Geometry: final body of the model. Coordinates: model frame, mm. Round coordinates to 2 decimals unless told otherwise and drop trailing zeros. Write item = value, one per line. Start each with the question number.
Item 1: Draft query along Y for faces 1 (the flat face through (215, 74, 0)), 2 (the cylindrical face through (422.98, 47.463, 1.127)). Return one class per face: pulls with the +Y half, pulls with the -Y half, needs draft (parallel to the pull), parting line crosses it, or undercut.
Item 2: First-contact query: pin 1 (5 mm diameter, centred on x = 167.64, y = 91.44, fed in from +Z). Flat tip, straight axial feed; report the tip coordinate or a pass-through.
Item 3: Section A-A (x = 105). Count the separate pieces of the cut face and the enclosed holes in it, plus the area to 3 significant figures.
Item 4: Line query: line 1 (Y direction, x = 269, z = 1.65); line 2 (Y direction, x = 89, z = 0.15); line 3 (X direction, y = 40, z = 0.3). Output: solid intervals per line, ascending. Write a range as from..to.
Autodesk Inventor part; units mm, degrees
ref_plane "YZ Plane" through (0, 0, 0) normal (1, 0, 0) x (0, 1, 0)
ref_plane "XZ Plane" through (0, 0, 0) normal (0, 1, 0) x (-1, 0, 0)
ref_plane "XY Plane" through (0, 0, 0) normal (0, 0, 1) x (1, 0, 0)
sketch "Sketch1" plane through (0, 0, 0) normal (0, 0, 1) x (1, 0, 0)
  line L0 (0, 0) -> (436.118, 0)
  line L1 (436.118, 0) -> (436.118, 101.6)
  line L2 (436.118, 101.6) -> (0, 101.6)
  line L3 (0, 101.6) -> (0, 0)
  circle A0 centre (12.7, 88.9) radius 3.3655
  circle A1 centre (12.7, 50.8) radius 3.3655
  circle A2 centre (12.7, 12.7) radius 3.3655
  circle A3 centre (423.418, 88.9) radius 3.3655
  circle A4 centre (423.418, 50.8) radius 3.3655
  circle A5 centre (423.418, 12.7) radius 3.3655
  circle A6 centre (218.059, 50.8) radius 20.32
  dimension "d0" = 436.118
  dimension "d1" = 101.6
  dimension "d2" = 6.731
  dimension "d3" = 12.7
  dimension "d4" = 12.7
  dimension "d7" = 38.1
  dimension "d10" = 410.718
  dimension "d13" = 12.7
  dimension "d24" = 40.64
  dimension "d25" = 50.8
  dimension "d26" = 218.059
extrude "Extrusion1" add sketch "Sketch1" along normal blind 2.286
sketch "Sketch2" plane through (0, 0, 2.286) normal (0, 0, 1) x (1, 0, 0)
  line L0 (0, 0) -> (436.118, 0)
  line L1 (82.55, 0) -> (133.35, 0)
  line L2 (31.75, 101.6) -> (184.15, 101.6)
  line L3 (133.35, 0) -> (184.15, 101.6)
  line L4 (31.75, 101.6) -> (82.55, 0)
  line L5 (97.1739, 7) -> (117.1739, 7)
  line L6 (117.1739, 7) -> (117.1739, 2)
  line L7 (117.1739, 2) -> (97.1739, 2)
  line L8 (97.1739, 2) -> (97.1739, 7)
  line L9 (133.35, 0) -> (133.35, 62.4863)
  line L10 (97.1739, 14) -> (117.1739, 14)
  line L11 (117.1739, 14) -> (117.1739, 9)
  line L12 (117.1739, 9) -> (97.1739, 9)
  line L13 (97.1739, 9) -> (97.1739, 14)
  line L14 (97.1739, 21) -> (117.1739, 21)
  line L15 (117.1739, 21) -> (117.1739, 16)
  line L16 (117.1739, 16) -> (97.1739, 16)
  line L17 (97.1739, 16) -> (97.1739, 21)
  line L18 (97.1739, 28) -> (117.1739, 28)
  line L19 (117.1739, 28) -> (117.1739, 23)
  line L20 (117.1739, 23) -> (97.1739, 23)
  line L21 (97.1739, 23) -> (97.1739, 28)
  line L22 (97.1739, 35) -> (117.1739, 35)
  line L23 (117.1739, 35) -> (117.1739, 30)
  line L24 (117.1739, 30) -> (97.1739, 30)
  line L25 (97.1739, 30) -> (97.1739, 35)
  line L26 (97.1739, 42) -> (117.1739, 42)
  line L27 (117.1739, 42) -> (117.1739, 37)
  line L28 (117.1739, 37) -> (97.1739, 37)
  line L29 (97.1739, 37) -> (97.1739, 42)
  circle A0 centre (126.2557, 6.2222) radius 3.1623
  circle A1 centre (126.2557, 28) radius 3.1623
  circle A2 centre (126.2557, 49.7778) radius 3.1623
  line L30 (107.95, 0) -> (107.95, -15.6085)
  circle A3 centre (89.6443, 49.7778) radius 3.1623
  circle A4 centre (89.6443, 6.2222) radius 3.1623
  circle A5 centre (89.6443, 28) radius 3.1623
  line L31 (117.1739, 44) -> (97.1739, 44)
  line L32 (97.1739, 44) -> (97.1739, 49)
  line L33 (117.1739, 49) -> (117.1739, 44)
  line L34 (97.1739, 49) -> (117.1739, 49)
  line L35 (117.1739, 51) -> (97.1739, 51)
  line L36 (97.1739, 51) -> (97.1739, 56)
  line L37 (97.1739, 56) -> (117.1739, 56)
  line L38 (117.1739, 56) -> (117.1739, 51)
  circle A6 centre (48.26, 91.44) radius 3.1623
  circle A7 centre (167.64, 91.44) radius 3.1623
  circle A8 centre (48.26, 10.16) radius 3.1623
  circle A9 centre (167.64, 10.16) radius 3.1623
  point P0 (0, 101.6)
  dimension "d37" = 50.8
  dimension "d38" = 152.4
  dimension "d39" = 101.6
  dimension "d40" = 50.8
  dimension "d41" = 20
  dimension "d42" = 5
  dimension "d43" = 2
  dimension "d44" = 7
  dimension "d45" = 6.3246
  dimension "d46" = 6.3246
  dimension "d47" = 6.3246
  dimension "d48" = 14
  dimension "d49" = 56
  dimension "d50" = 6.2222
  dimension "d51" = 6.2222
  dimension "d52" = 28
  dimension "d53" = 6.3246
  dimension "d54" = 6.3246
  dimension "d55" = 34.29
  dimension "d56" = 34.29
  dimension "d57" = 10.16
  dimension "d58" = 10.16
  dimension "d61" = 16.1761
  dimension "d62" = 31.75
  dimension "d112" = 9.0818
  dimension "d113" = 9.0818
  dimension "d114" = 9.0818
  dimension "d115" = 6.3246
  dimension "d116" = 10.16
  dimension "d117" = 34.29
  dimension "d118" = 6.3246
  dimension "d119" = 10.16
  dimension "d120" = 34.29
extrude "Extrusion2" cut sketch "Sketch2" against normal blind 2.286 contours L5 L6 L7 L8 | L10 L11 L12 L13 | L14 L15 L16 L17 | L18 L19 L20 L21 | L22 L23 L24 L25 | L26 L27 L28 L29 | A0 | A1 | A2 | A3 | A4 | A5 | L31 L32 L34 L33 | L35 L36 L37 L38 | A6 | A7 | A8 | A9
sketch "Sketch3" plane through (0, 0, 2.286) normal (0, 0, 1) x (1, 0, 0)
  circle A0 centre (126.2557, 49.7778) radius 3.1623
  line L0 (117.1739, 56) -> (117.1739, 51)
  line L1 (0, 0) -> (436.118, 0)
  line L2 (302.768, 0) -> (353.568, 0)
  line L3 (251.968, 101.6) -> (404.368, 101.6)
  line L4 (353.568, 0) -> (404.368, 101.6)
  line L5 (251.968, 101.6) -> (302.768, 0)
  line L6 (317.3919, 7) -> (337.3919, 7)
  line L7 (337.3919, 7) -> (337.3919, 2)
  line L8 (337.3919, 2) -> (317.3919, 2)
  line L9 (317.3919, 2) -> (317.3919, 7)
  line L10 (353.568, 0) -> (353.568, 62.4863)
  line L11 (317.3919, 14) -> (337.3919, 14)
  line L12 (337.3919, 14) -> (337.3919, 9)
  line L13 (337.3919, 9) -> (317.3919, 9)
  line L14 (317.3919, 9) -> (317.3919, 14)
  line L15 (317.3919, 21) -> (337.3919, 21)
  line L16 (337.3919, 21) -> (337.3919, 16)
  line L17 (337.3919, 16) -> (317.3919, 16)
  line L18 (317.3919, 16) -> (317.3919, 21)
  line L19 (317.3919, 28) -> (337.3919, 28)
  line L20 (337.3919, 28) -> (337.3919, 23)
  line L21 (337.3919, 23) -> (317.3919, 23)
  line L22 (317.3919, 23) -> (317.3919, 28)
  line L23 (317.3919, 35) -> (337.3919, 35)
  line L24 (337.3919, 35) -> (337.3919, 30)
  line L25 (337.3919, 30) -> (317.3919, 30)
  line L26 (317.3919, 30) -> (317.3919, 35)
  line L27 (317.3919, 42) -> (337.3919, 42)
  line L28 (337.3919, 42) -> (337.3919, 37)
  line L29 (337.3919, 37) -> (317.3919, 37)
  line L30 (317.3919, 37) -> (317.3919, 42)
  circle A1 centre (346.4737, 6.2222) radius 3.1623
  circle A2 centre (346.4737, 28) radius 3.1623
  circle A3 centre (346.4737, 49.7778) radius 3.1623
  line L31 (328.168, 0) -> (328.168, -15.6085)
  circle A4 centre (309.8623, 49.7778) radius 3.1623
  circle A5 centre (309.8623, 6.2222) radius 3.1623
  circle A6 centre (309.8623, 28) radius 3.1623
  line L32 (337.3919, 44) -> (317.3919, 44)
  line L33 (317.3919, 44) -> (317.3919, 49)
  line L34 (337.3919, 49) -> (337.3919, 44)
  line L35 (317.3919, 49) -> (337.3919, 49)
  line L36 (337.3919, 51) -> (317.3919, 51)
  line L37 (317.3919, 51) -> (317.3919, 56)
  line L38 (317.3919, 56) -> (337.3919, 56)
  line L39 (337.3919, 56) -> (337.3919, 51)
  circle A7 centre (268.478, 91.44) radius 3.1623
  circle A8 centre (387.858, 91.44) radius 3.1623
  circle A9 centre (268.478, 10.16) radius 3.1623
  circle A10 centre (387.858, 10.16) radius 3.1623
  point P0 (436.118, 101.6)
  dimension "d74" = 50.8
  dimension "d75" = 152.4
  dimension "d76" = 101.6
  dimension "d77" = 50.8
  dimension "d78" = 20
  dimension "d79" = 5
  dimension "d80" = 2
  dimension "d81" = 7
  dimension "d82" = 6.3246
  dimension "d83" = 6.3246
  dimension "d84" = 6.3246
  dimension "d85" = 14
  dimension "d86" = 56
  dimension "d87" = 6.2222
  dimension "d88" = 6.2222
  dimension "d89" = 28
  dimension "d90" = 6.3246
  dimension "d91" = 6.3246
  dimension "d92" = 34.29
  dimension "d93" = 34.29
  dimension "d94" = 10.16
  dimension "d95" = 10.16
  dimension "d98" = 16.1761
  dimension "d99" = 31.75
  dimension "d100" = 9.0818
  dimension "d101" = 9.0818
  dimension "d102" = 9.0818
  dimension "d103" = 9.0818
  dimension "d104" = 6.3246
  dimension "d105" = 10.16
  dimension "d106" = 34.29
  dimension "d107" = 6.3246
  dimension "d108" = 10.16
  dimension "d109" = 34.29
extrude "Extrusion3" cut sketch "Sketch3" against normal blind 6.3246 contours L6 L7 L8 L9 | L11 L12 L13 L14 | L15 L16 L17 L18 | L19 L20 L21 L22 | L23 L24 L25 L26 | L27 L28 L29 L30 | A1 | A2 | A3 | A4 | A5 | A6 | L32 L33 L35 L34 | L36 L37 L38 L39 | A7 | A8 | A9 | A10
equation "\"d26\" = 0.5 * d0"
equation "\"d46\" = d45"
equation "\"d47\" = d46"
equation "\"d50\" = 0.111111 * d49"
equation "\"d51\" = d50"
equation "\"d52\" = 0.5 * d49"
equation "\"d56\" = d55"
equation "\"d58\" = d57"
equation "\"d113\" = d112"
equation "\"d114\" = d112"
equation "\"d116\" = d57"
equation "\"d117\" = d56"
equation "\"d119\" = d58"
equation "\"d120\" = d55"
equation "\"d83\" = d82"
equation "\"d84\" = d83"
equation "\"d87\" = 0.111111 * d86"
equation "\"d88\" = d87"
equation "\"d89\" = 0.5 * d86"
equation "\"d93\" = d92"
equation "\"d95\" = d94"
equation "\"d102\" = d100"
equation "\"d103\" = d100"
equation "\"d105\" = d94"
equation "\"d106\" = d93"
equation "\"d108\" = d95"
equation "\"d109\" = d92"
equation "\"d110\" = d83"
properties part number "elevbackpltblt"
Taken from the geometry:
q1.face_1 = needs draft
q1.face_2 = undercut
q2.pin_1 = through
q3.separate_pieces = 9
q3.enclosed_holes = 0
q3.area = 141 mm^2
q4.line_1 = 0..7.04, 13.28..88.32, 94.56..101.6
q4.line_2 = 0..3.13, 9.32..24.9, 31.1..46.68, 52.87..101.6
q4.line_3 = 0..97.17, 117.17..200.85, 235.27..317.39, 337.39..436.12
